Part print with two shaded views. Sizes in mm from the minimum x, y, z corner. A direction names the side the tool comes from. Coordinates: 2 decimals unless noted, no trailing zeros. Loops run counter-clockwise (first coordinate to the right, second up) from the corner with the lowest first, then second, coordinate; pieces in that order, holes last. Notation, with made-up numbers: (13, -30.75) -> (60, -30.75) arc R34 cw to (60, 5.25) -> close; hole circle Ø11 at (81.25, -20.5). An arc over 180 degrees is marked (long way). Return JSON: item names as keys, results as strings. Group by question number.
(1) Saw through at C-C on y = 15.75. Write the cut outline in (x, z) (1 decimal), then the cut area to 3 significant figures.
(2) Mould opens along X. For the marked faces 1, 2 and 3 say: pulls with the +X half, pulls with the -X half, needs draft (parallel to the pull), parting line crosses it, or undercut.
(3) Tool access for the marked faces 4 and 5: list every direction of +Z, -Z, +X, -X, +Y, -Y with a clear straight run to the whole face (end or side of a thin tool).
(4) Saw through at A-A on y = 2.5. Write the cut outline in (x, z) (1 decimal).
(5) Saw through at B-B on z = 2.75. Write the cut outline in (x, y) (1 decimal), then the cut area to 3 significant figures.
(6) Flat gauge pins, fed straight in: pin 1 Ø6 at (x, z) = (3.5, 9.5) entering from -Y; pin 2 Ø1.5 at (x, z) = (3.5, 11.5) entering from +Y; pin 3 Ø4 at (x, y) = (9.5, 3.5) entering from -Z (1 decimal). Where does each tip first touch, or does it go through?
(7) Probe L1, parallel to X at y = 2.25, z = 8.75 (1 decimal); L2, parallel to Z at x = 6, y = 11; L3, parallel to Z at x = 10.25, y = 6. List the from-to ranges inside material, lowest first.
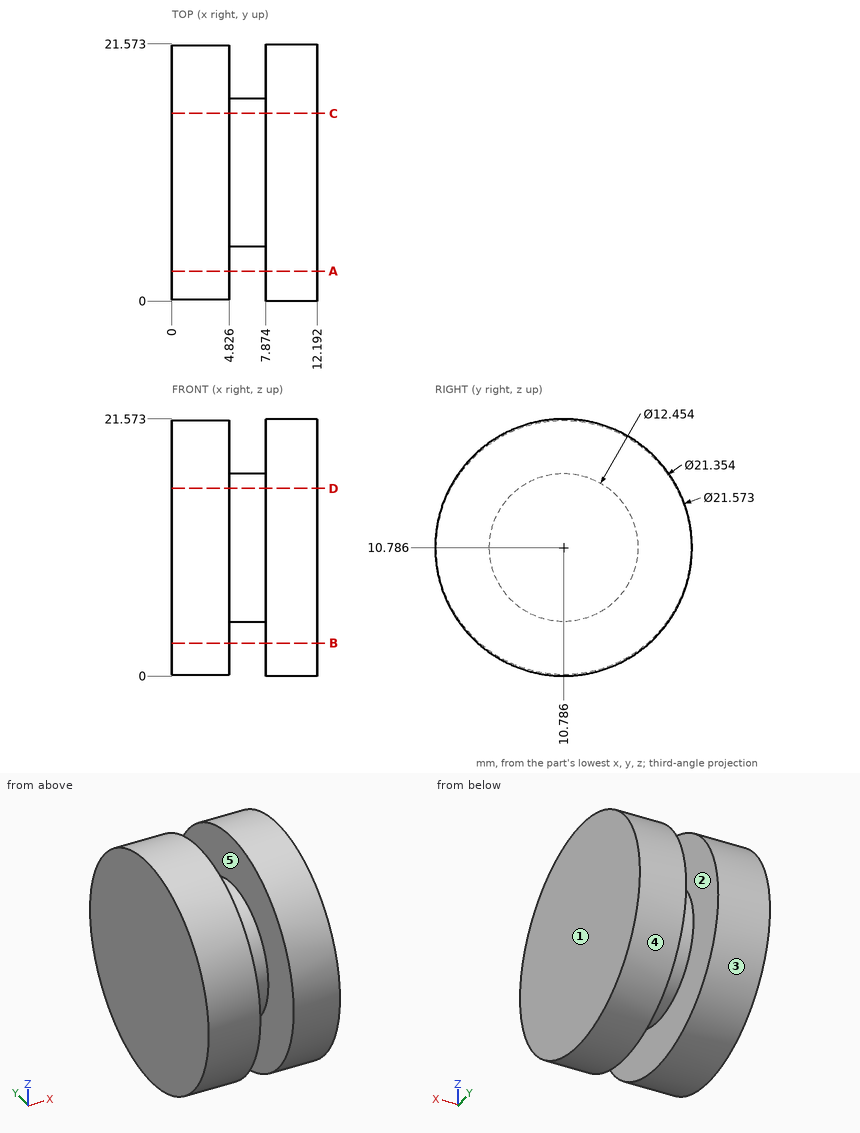
Geometry results:
{
 "1": {"outline": "(0, 1.3) -> (4.8, 1.3) -> (4.8, 7) -> (7.9, 7) -> (7.9, 1.2) -> (12.2, 1.2) -> (12.2, 20.4) -> (7.9, 20.4) -> (7.9, 14.5) -> (4.8, 14.5) -> (4.8, 20.2) -> (0, 20.2) -> close", "area": "197 mm²"},
 "2": {"face 1": "pulls with the +X half", "face 2": "undercut", "face 3": "needs draft"},
 "3": {"face 4": "+X, -X", "face 5": "none"},
 "4": {"outline": "(0, 4.1) -> (4.8, 4.1) -> (4.8, 17.5) -> (0, 17.5) -> close; (7.9, 3.9) -> (12.2, 3.9) -> (12.2, 17.7) -> (7.9, 17.7) -> close"},
 "5": {"outline": "(0, 3.8) -> (4.8, 3.8) -> (4.8, 17.8) -> (0, 17.8) -> close; (7.9, 3.6) -> (12.2, 3.6) -> (12.2, 18) -> (7.9, 18) -> close", "area": "130 mm²"},
 "6": {"pin 1": "y = 0.11", "pin 2": "y = 21.46", "pin 3": "z = 1.4"},
 "7": {"L1": "0 to 4.8, 7.9 to 12.2", "L2": "4.56 to 17.01", "L3": "1.12 to 20.45"}
}
